Read the model definition and answer for the solid it produces. Units are mm, in the model's axes. A direction names the side the tool comes from. Coordinates: 2 decimals unless noted, no trailing zeros. Loops run counter-clockwise (first coordinate to the right, second up) from the corner with the lowest first, then second, coordinate; pieces in that order, holes last. Notation, with made-up numbers: (-2, -31.75) -> (28, -31.75) arc R21 cw to (28, -23.75) -> close; hole circle Ø4 at (24.5, 19). An arc over 180 degrees is marked (long way). One line per question, with ' | ' between items. Start each with the question number.
```python
from build123d import *

# Parameters (mm, degrees)
SKETCH1_W           = 40
SKETCH1_H           = 240
BOSS_EXTRUDE2_DEPTH = 2
SKETCH2_W           = 40
SKETCH2_H           = 240
SKETCH2_W_2         = 36
SKETCH2_H_2         = 236
BOSS_EXTRUDE4_DEPTH = 45
SKETCH3_W           = 14
SKETCH3_H           = 14
BOSS_EXTRUDE5_DEPTH = 45
SKETCH4_R           = 1.75
CUT_EXTRUDE1_DEPTH  = 90
SKETCH5_R           = 3.5
CUT_EXTRUDE2_DEPTH  = 45
SKETCH6_W           = 20
SKETCH6_H           = 10
CUT_EXTRUDE3_DEPTH  = 10
FILLET3_R           = 10
FILLET4_R           = 10
SKETCH7_W           = 75
SKETCH7_H           = 47
BOSS_EXTRUDE6_DEPTH = 45
SKETCH8_W           = 45
SKETCH8_H           = 71
CUT_EXTRUDE4_DEPTH  = 45
SKETCH9_W           = 36
SKETCH9_H           = 4
CUT_EXTRUDE5_DEPTH  = 45


with BuildPart() as part:
    # Sketch1 → Boss-Extrude2 (new body)
    with BuildSketch(Plane(origin=(0, 0, 0), x_dir=(1, 0, 0), z_dir=(0, 1, 0))):
        Rectangle(SKETCH1_W, SKETCH1_H)
    extrude(amount=BOSS_EXTRUDE2_DEPTH)

    # Sketch2 → Boss-Extrude4 (add)
    with BuildSketch(Plane(origin=(0, 2, 0), x_dir=(1, 0, 0), z_dir=(0, 1, 0))):
        Rectangle(SKETCH2_W, SKETCH2_H)
        Rectangle(SKETCH2_W_2, SKETCH2_H_2, mode=Mode.SUBTRACT)
    extrude(amount=BOSS_EXTRUDE4_DEPTH)

    # Sketch3 → Boss-Extrude5 (add)
    with BuildSketch(Plane(origin=(0, 2, 0), x_dir=(1, 0, 0), z_dir=(0, 1, 0))):
        with Locations((-11, 111)):
            Rectangle(SKETCH3_W, SKETCH3_H)
        with Locations((11, 111)):
            Rectangle(SKETCH3_W, SKETCH3_H)
        with Locations((-11, -111)):
            Rectangle(SKETCH3_W, SKETCH3_H)
        with Locations((11, -111)):
            Rectangle(SKETCH3_W, SKETCH3_H)
    extrude(amount=BOSS_EXTRUDE5_DEPTH)

    # Sketch4 → Cut-Extrude1 (cut)
    with BuildSketch(Plane(origin=(0, 0, 0), x_dir=(-1, 0, 0), z_dir=(0, -1, 0))):
        with Locations(Location((12, -112, 0), (0, 0, 90))):
            Circle(SKETCH4_R)
        with Locations(Location((-13, -112, 0), (0, 0, 90))):
            Circle(SKETCH4_R)
        with Locations(Location((12, 112, 0), (0, 0, 90))):
            Circle(SKETCH4_R)
        with Locations(Location((-13, 112, 0), (0, 0, 90))):
            Circle(SKETCH4_R)
    extrude(amount=-CUT_EXTRUDE1_DEPTH, mode=Mode.SUBTRACT)

    # Sketch5 → Cut-Extrude2 (cut)
    with BuildSketch(Plane(origin=(0, 0, 0), x_dir=(-1, 0, 0), z_dir=(0, -1, 0))):
        with Locations(Location((12, -112, 0), (0, 0, 90))):
            Circle(SKETCH5_R)
        with Locations(Location((-13, -112, 0), (0, 0, 90))):
            Circle(SKETCH5_R)
        with Locations(Location((12, 112, 0), (0, 0, 90))):
            Circle(SKETCH5_R)
        with Locations(Location((-13, 112, 0), (0, 0, 90))):
            Circle(SKETCH5_R)
    extrude(amount=-CUT_EXTRUDE2_DEPTH, mode=Mode.SUBTRACT)

    # Sketch6 → Cut-Extrude3 (cut)
    with BuildSketch(Plane(origin=(20, 0, 0), x_dir=(0, 0, -1), z_dir=(1, 0, 0))):
        with Locations((0, 42)):
            Rectangle(SKETCH6_W, SKETCH6_H)
    extrude(amount=-CUT_EXTRUDE3_DEPTH, mode=Mode.SUBTRACT)

    # Fillet3
    fillet3_edges = [part.edges().sort_by_distance(p)[0] for p in [
        (-20, 23.5, -120),
    ]]
    fillet(fillet3_edges, radius=FILLET3_R)

    # Fillet4
    fillet4_edges = [part.edges().sort_by_distance(p)[0] for p in [
        (-20, 23.5, 120),
    ]]
    fillet(fillet4_edges, radius=FILLET4_R)

    # Sketch7 → Boss-Extrude6 (add)
    with BuildSketch(Plane(origin=(20, 0, 0), x_dir=(0, 0, -1), z_dir=(1, 0, 0))):
        with Locations((82.5, 23.5)):
            Rectangle(SKETCH7_W, SKETCH7_H)
    extrude(amount=BOSS_EXTRUDE6_DEPTH)

    # Sketch8 → Cut-Extrude4 (cut)
    with BuildSketch(Plane(origin=(0, 47, 0), x_dir=(1, 0, 0), z_dir=(0, 1, 0))):
        with Locations((40.5, 82.5)):
            Rectangle(SKETCH8_W, SKETCH8_H)
    extrude(amount=-CUT_EXTRUDE4_DEPTH, mode=Mode.SUBTRACT)

    # Sketch9 → Cut-Extrude5 (cut)
    with BuildSketch(Plane(origin=(0, 47, 0), x_dir=(1, 0, 0), z_dir=(0, 1, 0))):
        with Locations((0, 106)):
            Rectangle(SKETCH9_W, SKETCH9_H)
    extrude(amount=-CUT_EXTRUDE5_DEPTH, mode=Mode.SUBTRACT)


solid = part.part
```
(1) Section A-A on y = 24 is taken. Write down the section's boundary in (x, z).
(2) Determine the mould class of faces 6 (the cylindrical face through (-17.15, 23.83, 116.99)), 7 (the flat face through (-13, 45, -110)), 8 (the flat face through (27, 23, -120)), 9 (the cylindrical face through (11.659, 22.185, 108.767)) for opening direction Z: +Z half, -Z half, draft (parallel to the pull), parting line (faces both ways), or undercut.
(3) Section B-B on z = 2 is taken. Write down the section's boundary in (x, y).
(4) A tool of negligible diameter and unlimited length cuts with its end or side. For faces 1 (the flat face through (11, 25, -108)), 2 (the flat face through (42, 23, -45)), 3 (the flat face through (-13, 45, 114)), 4 (the flat face through (65, 24, -82)), 5 (the flat face through (-20, 23, 2)), from which of +Z, -Z, +X, -X, +Y, -Y can it reach the whole face along a straight path? Write none if from no direction.
(5) Section C-C on x = 49 is taken. Write down the section's boundary in (y, z), plus the area to 3 significant figures.
(6) Find the intervals of material crossed by probe 1 along X at (y, z) = (23.5, -100); probe 2 along Z at (x, y) = (7, 38.5); probe 3 along Z at (x, y) = (20.5, 10), in increasing order. Write a range as from..to.
(7) Each of these flat-tipped pins is pushed along its axis until it touches: pin 1 Ø2 at (x, z) = (-10.5, 76) entering from +Y; pin 2 Ø3.5 at (x, z) = (11.5, -112.5) entering from -Y; pin 3 Ø4.5 at (x, z) = (-12, 112) entering from +Y; pin 4 Ø1.6 at (x, z) = (19, 3) entering from +Y. Where does it stop, or does it pass through?
Working result:
1) outline: (-20, -110) arc R10 ccw to (-10, -120) -> (65, -120) -> (65, -45) -> (20, -45) -> (20, 120) -> (-10, 120) arc R10 ccw to (-20, 110) -> close; hole (-18, -108) -> (-4, -108) -> (-4, -118) -> (4, -118) -> (4, -108) -> (18, -108) -> (18, -118) -> (63, -118) -> (63, -47) -> (18, -47) -> (18, 104) -> (4, 104) -> (4, 118) -> (-4, 118) -> (-4, 104) -> (-18, 104) -> close; hole circle Ø7 at (-12, -112); hole circle Ø7 at (-12, 112); hole circle Ø7 at (13, -112); hole circle Ø7 at (13, 112)
2) face 6: +Z half | face 7: undercut | face 8: -Z half | face 9: undercut
3) outline: (-20, 0) -> (20, 0) -> (20, 37) -> (18, 37) -> (18, 2) -> (-18, 2) -> (-18, 47) -> (-20, 47) -> close
4) face 1: +Y | face 2: +Z, +X, +Y, -Y | face 3: -Y | face 4: +Z, -Z, +X, +Y, -Y | face 5: +Z, -Z, -X, +Y, -Y
5) outline: (0, -120) -> (47, -120) -> (47, -118) -> (2, -118) -> (2, -47) -> (47, -47) -> (47, -45) -> (0, -45) -> close | area: 330 mm2
6) probe 1: x = -20..-18, 63..65 | probe 2: z = -120..-108, 104..120 | probe 3: z = -120..-118, -47..-45
7) pin 1: stops at y = 2 | pin 2: stops at y = 45 | pin 3: stops at y = 47 | pin 4: stops at y = 37
